Answer from the drawing. Dimensions are ordinates in mm from the lowest x, y and z of the part. A direction names the side the tool comes from. Coordinates: 2 decimals unless noted, no trailing zeros. Order: outer loops, then holes, each group sorted by start corner. A loop starts at its lowest first (then second) coordinate and runs counter-clockwise, first axis right, second up. Notation, with made-up numbers: (70.5, -21.5) - (95.5, -21.5) arc R15 ccw to (95.5, -11.5) - close; hole circle Ø5 at (-39.5, -35.75). An arc over 180 degrees is marked (long way). Use a Markdown table: item, result. Add a question column.
Item 1: For the marked faces 1, 2, 3, 4 and 5, determine the directions among +Z, -Z, +X, -X, +Y, -Y from which every point of the face is accessible in a straight line to the end or side of a thin tool.
Item 2: The part is cut by section A-A, the plane x = 3.75. Give the vertices of the cut face in (y, z), then the cut area to 3 significant figures.
Item 3: The part is cut by section D-D, the plane z = 2.5. Give the vertices of the cut face in (x, y), then the cut area to 3 significant figures.
Item 4: Flat-ended cylindrical pins translate along their axes: P1, Ø3, axis at x = 7.5, y = 3, coming from the +Z side; P2, Ø1.5, axis at y = 8.5, z = 5.5, coming from the +X side; P3, Ø2, axis at y = 4, z = 3.5, coming from the -X side. Find the tip coordinate at first contact, or state that the pin passes through.
Item 5: The part is cut by section B-B, the plane z = 3.75. Give the vertices of the cut face in (x, y).
Item 6: The part is cut by section C-C, the plane y = 4. Give the vertices of the cut face in (x, z).
Item 7: Find the intervals of material crossed by line 1 along Z through (x, y) = (6.75, 13); line 2 along Y through (x, z) = (7.5, 1.75); line 3 along Y through (x, z) = (2, 5), in increasing order.
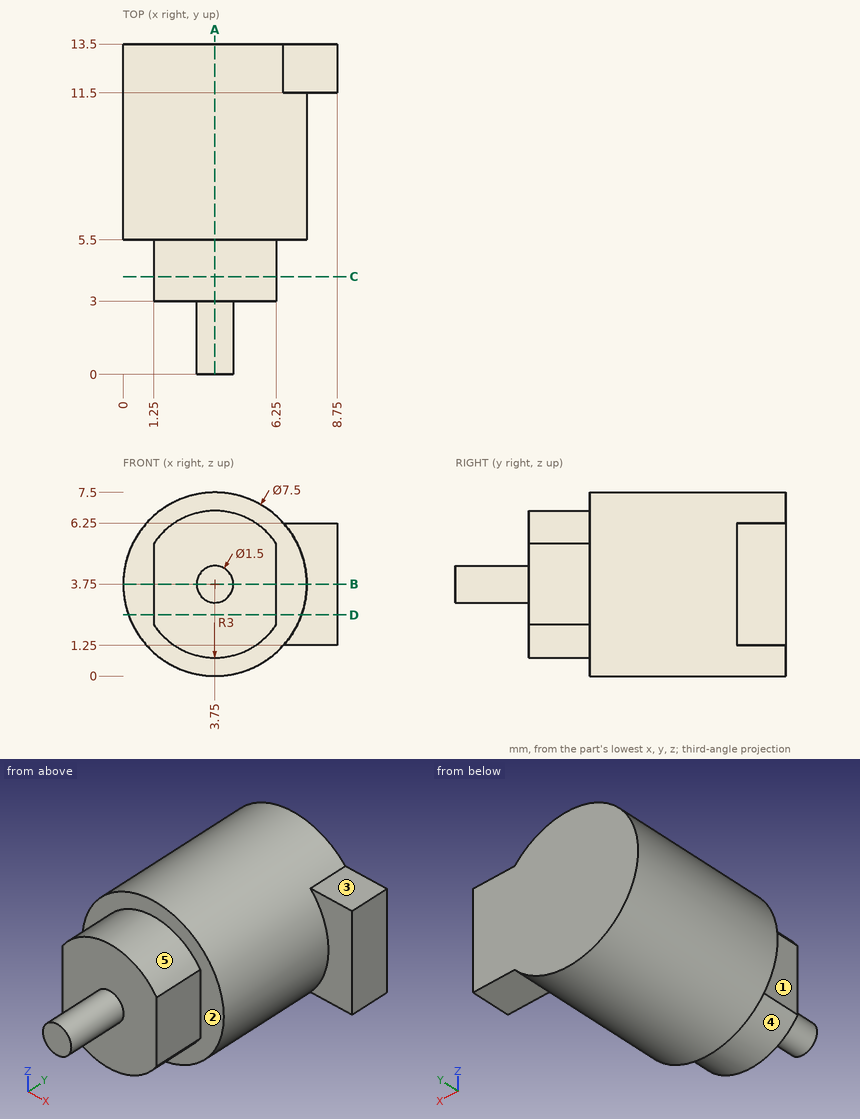
Solution:
| question | item | result |
|---|---|---|
| 1 | face 1 | +Z, -Z, -X, -Y |
| 1 | face 2 | -Y |
| 1 | face 3 | +Z, +X, +Y, -Y |
| 1 | face 4 | -Z, -Y |
| 1 | face 5 | +Z, -Y |
| 2 | outline | (0, 3) - (3, 3) - (3, 0.75) - (5.5, 0.75) - (5.5, 0) - (13.5, 0) - (13.5, 7.5) - (5.5, 7.5) - (5.5, 6.75) - (3, 6.75) - (3, 4.5) - (0, 4.5) - close |
| 2 | area | 79.5 mm2 |
| 3 | outline | (0.21, 5.5) - (1.25, 5.5) - (1.25, 3) - (6.25, 3) - (6.25, 5.5) - (7.29, 5.5) - (7.29, 11.5) - (8.75, 11.5) - (8.75, 13.5) - (0.21, 13.5) - close |
| 3 | area | 72.0 mm2 |
| 4 | P1 | stops at z = 5.73 |
| 4 | P2 | stops at x = 7.36 |
| 4 | P3 | stops at x = 1.25 |
| 5 | outline | (0, 5.5) - (1.25, 5.5) - (1.25, 3) - (3, 3) - (3, 0) - (4.5, 0) - (4.5, 3) - (6.25, 3) - (6.25, 5.5) - (7.5, 5.5) - (7.5, 11.5) - (8.75, 11.5) - (8.75, 13.5) - (0, 13.5) - close |
| 6 | outline | (1.25, 2.09) arc R3 ccw to (6.25, 2.09) - (6.25, 5.41) arc R3 ccw to (1.25, 5.41) - close |
| 7 | line 1 | z = 1.25 to 6.25 |
| 7 | line 2 | y = 11.5 to 13.5 |
| 7 | line 3 | y = 3 to 13.5 |
